Build history of the part. All positions in model axes, mm. Round coordinates to 2 decimals unless told otherwise and drop trailing zeros. Write each loop counter-clockwise with the first axis right and the second up, starting at its lowest first coordinate (ties: lowest second). Pieces come first, ordered by that corner, then holes. Notation, with made-up numbers: (66, 84) -> (99, 84) arc R9 ccw to (99, 90) -> close; hole circle Ø10 at (58, -23). An arc over 180 degrees is marked (long way). Answer as CSV lines item,"result".
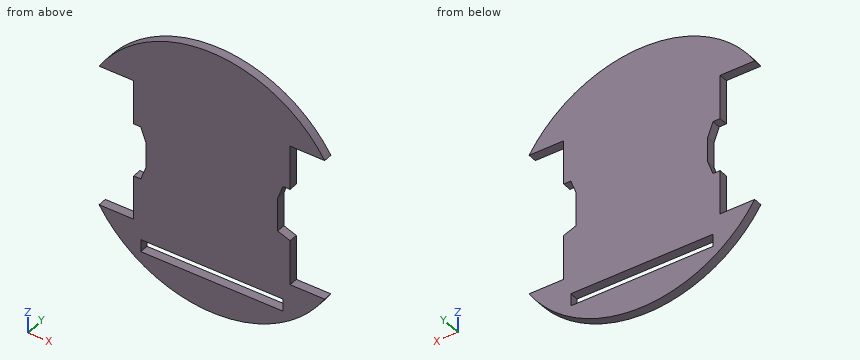
from build123d import *

# Parameters (mm, degrees)
SKETCH1_W           = 80
SKETCH1_H           = 7
BOSS_EXTRUDE1_DEPTH = 5
CHAMFER1_SIZE       = 8
CHAMFER1_SIZE_2     = 3


with BuildPart() as part:
    # Sketch1 → Boss-Extrude1 (new body)
    with BuildSketch(Plane(origin=(0, 0, 0), x_dir=(1, 0, 0), z_dir=(0, 1, 0))):
        with BuildLine():
            Line((-44, -40), (-44, -15))
            Line((-44, -15), (-37, -15))
            Line((-37, -15), (-37, 15))
            Line((-37, 15), (-44, 15))
            Line((-44, 15), (-44, 40))
            Line((-44, 40), (-63.442887702, 40))
            ThreePointArc((-63.442887702, 40), (0, 75), (63.442887702, 40))
            Line((63.442887702, 40), (44, 40))
            Line((44, 40), (44, 15))
            Line((44, 15), (37, 15))
            Line((37, 15), (37, -15))
            Line((37, -15), (44, -15))
            Line((44, -15), (44, -40))
            Line((44, -40), (63.442887702, -40))
            ThreePointArc((63.442887702, -40), (0, -75), (-63.442887702, -40))
            Line((-63.442887702, -40), (-44, -40))
        make_face()
        with Locations((0, 53.524444958)):
            Rectangle(SKETCH1_W, SKETCH1_H, mode=Mode.SUBTRACT)
    extrude(amount=BOSS_EXTRUDE1_DEPTH)

    # Chamfer1
    # the kernel refuses this chamfer: 8, 3 mm, written as the material it adds along each edge
    with BuildSketch(Plane(origin=(37, 0, 15), x_dir=(-0.013536660009854304, 0, -0.9999083752203387), z_dir=(0, 1, 0)), Plane(origin=(-37, 0, -15), x_dir=(0.013536660009854304, 0, 0.9999083752203387), z_dir=(0, 1, 0))) as chamfer1_piece_1:
        Polygon((CHAMFER1_SIZE * 0.99990837522, -CHAMFER1_SIZE * 0.0135366600099), (-CHAMFER1_SIZE_2 * 0.0135366600099, -CHAMFER1_SIZE_2 * 0.99990837522), (0, 0), align=None)
    extrude(amount=5)
    with BuildSketch(Plane(origin=(37, 0, -15), x_dir=(0.9999083752203387, 0, -0.013536660009854514), z_dir=(0, 1, 0))) as chamfer1_piece_2_section:
        Polygon((CHAMFER1_SIZE * 0.99990837522, -CHAMFER1_SIZE * 0.0135366600099), (-CHAMFER1_SIZE_2 * 0.0135366600099, -CHAMFER1_SIZE_2 * 0.99990837522), (0, 0), align=None)
    chamfer1_piece_2 = extrude(amount=5, mode=Mode.PRIVATE)
    chamfer1_piece_2 = split(chamfer1_piece_2, bisect_by=Plane(origin=(44, 2.5, -14.03968053), z_dir=(-1, 0, 0)), keep=Keep.TOP, mode=Mode.PRIVATE)
    add(chamfer1_piece_2)
    with BuildSketch(Plane(origin=(-37, 0, 15), x_dir=(-0.9953980532473654, 0, 0.09582648689874379), z_dir=(0, 1, 0))) as chamfer1_piece_3:
        Polygon((CHAMFER1_SIZE_2 * 0.995398053247, -CHAMFER1_SIZE_2 * 0.0958264868987), (-CHAMFER1_SIZE * 0.0958264868987, -CHAMFER1_SIZE * 0.995398053247), (0, 0), align=None)
    extrude(amount=5)


solid = part.part
1. Cut at C-C, the plane z = -9. Write the cut outline in (x, y).
Results found:
outline,"(-37.75, 0) -> (37, 0) -> (37, 5) -> (-37.75, 5) -> close"
2. Probe line 1 along Z through (x, y) = (-30, 2.25); line 2 along Z through (x, y) = (-21, 2.2); line 3 along X through (y, z) = (3.8, -22). List the from-to ranges inside material, lowest first.
Results found:
line 1,"z = -68.74 to -57.02, -50.02 to 68.74"
line 2,"z = -72 to -57.02, -50.02 to 72"
line 3,"x = -44 to 44"
3. Cut at A-A, the plane y = 2.9. Write the cut outline in (x, z) (3 decimals).
Results found:
outline,"(-63.443, -40) arc R75 ccw to (63.443, -40) -> (44, -40) -> (44, -14.625) -> (37, -12) -> (37, 7) -> (40, 15) -> (44, 15) -> (44, 40) -> (63.443, 40) arc R75 ccw to (-63.443, 40) -> (-44, 40) -> (-44, 15) -> (-40, 15) -> (-37, 7) -> (-37, -7) -> (-40, -15) -> (-44, -15) -> (-44, -40) -> close; hole (-40, -57.024) -> (40, -57.024) -> (40, -50.024) -> (-40, -50.024) -> close"
4. Cut at D-D, the plane x = 31.5. Write the cut outline in (y, z).
Results found:
outline,"(0, -68.06) -> (5, -68.06) -> (5, -57.02) -> (0, -57.02) -> close; (0, -50.02) -> (5, -50.02) -> (5, 68.06) -> (0, 68.06) -> close"
5. Cut at B-B, the plane x = 49. Write the cut outline in (y, z), then the cut area to 3 significant figures.
Results found:
outline,"(0, -56.78) -> (5, -56.78) -> (5, -40) -> (0, -40) -> close; (0, 40) -> (5, 40) -> (5, 56.78) -> (0, 56.78) -> close"
area,"168 mm2"
6. Drop flat-ended pins along their axis: pin 1 Ø2.5 at (y, z) = (2, -53.5) entering from -X; pin 2 Ø2.5 at (y, z) = (1.5, 25.5) entering from +X; pin 3 Ø1.5 at (y, z) = (1.5, -25) entering from -X; pin 4 Ø5 at (x, z) = (-5, -28) entering from -Y. Give the stop position or say it passes through.
Results found:
pin 1,"stops at x = -53.8"
pin 2,"stops at x = 44"
pin 3,"stops at x = -44"
pin 4,"stops at y = 0"
